Verification items for the finished model (mm, model axes). A direction names the side the tool comes from. Give positions to 0.01 mm unless a question says otherwise; leave off trailing zeros. Order: outer loops, then holes, each group sorted by start corner. A loop starts at its lowest first (then second) coordinate and runs counter-clockwise, first axis right, second up. Notation, with made-up numbers: (1.5, -38) -> (17.5, -38) arc R15 ccw to (17.5, -19) -> close; hole circle Ø8 at (-15.5, 12). An arc over 180 degrees is marked (long way). Return JSON: item names as keys, results as strings. Group by question number.
(1) Depth check by flat-ended pin: pin 1 Ø0.8 at (x, z) = (-50.5, -1.5) entering from -Y; pin 2 Ø12 at (x, y) = (-7.5, 13.5) entering from -Z; pin 3 Ø1.5 at (x, z) = (15, 1.5) entering from +Y. Enter the tip coordinate at first touch or a pass-through.
(2) Cross-section at A-A on z = -1.3. Enter the section's corners in (x, y).
(3) Thickness scan on line 1 along Z through (x, y) = (12, -8); line 2 along Y through (x, z) = (40, 0.3); line 3 along Y through (x, z) = (40, 2). Record the ranges inside material, lowest first.
(4) Tool access check on faces 1 (the face through (-50, -5, -1)), 2 (the face through (42, -2, 1.5)), 3 (the face through (-50, 5, -1)), 4 (the face through (-41, 0, -2)). Record the directions out of +Z, -Z, +X, -X, +Y, -Y that give a thin tool (end or side, any length) a straight path to the whole face; none if there is none.
(5) Release check for a two-part mould opening along X. For faces 5 (the face through (35, 0, 2)), 6 (the face through (-51, 0, -2.5)), 7 (the face through (-60, 0, -1)) record: pulls with the +X half, pulls with the -X half, needs draft (parallel to the pull), parting line crosses it, or undercut.
from build123d import *

# Parameters (mm, degrees)
F0_R     = 5
F1_DEPTH = 3
F0_R_2   = 2.5
F2_DEPTH = 1.5
F3_DEPTH = 2.5
F4_R     = 2.49999
F5_R     = 2


# Not quite as in the source:
# - a fillet or chamfer is up to 0.001 mm smaller than in the source, because OpenCascade refuses the exact size


with BuildPart() as f1:
    # F0 (on Top) → F1 (new body)
    with BuildSketch(Plane.XY):
        with BuildLine():
            ThreePointArc((-49.7493718553, -5), (2.503138753, -49.9373036555), (50, 0))
            ThreePointArc((50, 0), (2.503138753, 49.9373036555), (-49.7493718553, 5))
            Line((-49.7493718553, 5), (-40, 5))
            Line((-40, 5), (-40, -5))
            Line((-40, -5), (-49.7493718553, -5))
        make_face()
        with Locations((40, 0)):
            Circle(F0_R, mode=Mode.SUBTRACT)
        with BuildLine():
            Line((-40, 5), (-49.7493718553, 5))
            ThreePointArc((-49.7493718553, 5), (-50, 0), (-49.7493718553, -5))
            Line((-49.7493718553, -5), (-40, -5))
            Line((-40, -5), (-40, 5))
        make_face()
    extrude(amount=F1_DEPTH)

    # F0 (on Top) → F2 (join)
    with BuildSketch(Plane.XY):
        with Locations((40, 0)):
            Circle(F0_R)
        with Locations((40, 0)):
            Circle(F0_R_2, mode=Mode.SUBTRACT)
    extrude(amount=F2_DEPTH)

    # F0 (on Top) → F3 (join)
    with BuildSketch(Plane.XY):
        with BuildLine():
            ThreePointArc((-49.7493718553, -5), (-50, 0), (-49.7493718553, 5))
            Line((-49.7493718553, 5), (-60, 5))
            Line((-60, 5), (-60, -5))
            Line((-60, -5), (-49.7493718553, -5))
        make_face()
        with BuildLine():
            Line((-40, 5), (-49.7493718553, 5))
            ThreePointArc((-49.7493718553, 5), (-50, 0), (-49.7493718553, -5))
            Line((-49.7493718553, -5), (-40, -5))
            Line((-40, -5), (-40, 5))
        make_face()
    extrude(amount=-F3_DEPTH)

    # F4 (radius 2.5 in the source; OpenCascade refuses exactly that, so slightly less here)
    f4_edges = [f1.edges().sort_by_distance(p)[0] for p in [
        (-40, 0, -2.5),
    ]]
    fillet(f4_edges, radius=F4_R)

    # F5
    f5_edges = [f1.edges().sort_by_distance(p)[0] for p in [
        (-50, 0, 3),
    ]]
    fillet(f5_edges, radius=F5_R)


solid = f1.part
Verdict:
{
 "1": {"pin 1": "y = -5", "pin 2": "z = 0", "pin 3": "y = 47.9"},
 "2": {"outline": "(-60, -5) -> (-40.36, -5) -> (-40.36, 5) -> (-60, 5) -> close"},
 "3": {"line 1": "0 to 3", "line 2": "-30 to -2.5, 2.5 to 30", "line 3": "-29.55 to -5, 5 to 29.55"},
 "4": {"face 1": "-Z, +X, -X, -Y", "face 2": "+Z", "face 3": "-Z, +X, -X, +Y", "face 4": "-Z, +X, +Y, -Y"},
 "5": {"face 5": "undercut", "face 6": "needs draft", "face 7": "pulls with the -X half"}
}
